Can you work these out from the model? Positions are in its coordinate system, mm. A direction names the side the tool comes from. Coordinates: 2 decimals unless noted, no trailing zeros. Order: outer loops, then holes, each group sorted by start corner. A loop starts at its lowest first (then second) coordinate and runs counter-clockwise, first axis right, second up. Notation, with made-up numbers: (57.5, 79) -> (102.5, 79) arc R35 ccw to (102.5, 111) -> close; hole circle Ø11 at (-24.75, 86). An arc over 180 degrees is marked (long way). Write item = value, one per line.
```python
from build123d import *

# Parameters (mm, degrees)
SKETCH1_W           = 76.2
SKETCH1_H           = 25.4
SKETCH1_W_2         = 70.104
SKETCH1_H_2         = 19.304
BOSS_EXTRUDE1_DEPTH = 200
SKETCH3_W           = 76.2
SKETCH3_H           = 25.4
SKETCH3_W_2         = 70.104
SKETCH3_H_2         = 19.304
BOSS_EXTRUDE2_DEPTH = 38.1
CUT_EXTRUDE1_DEPTH  = 77.2
CUT_EXTRUDE2_START  = 13.832764
SKETCH6_R           = 38.1
CUT_EXTRUDE2_DEPTH  = 83.124802


with BuildPart() as part:
    # Sketch1 → Boss-Extrude1 (new body)
    with BuildSketch(Plane(origin=(0, 0, 0), x_dir=(1, 0, 0), z_dir=(0, 1, 0))):
        Rectangle(SKETCH1_W, SKETCH1_H)
        Rectangle(SKETCH1_W_2, SKETCH1_H_2, mode=Mode.SUBTRACT)
    extrude(amount=BOSS_EXTRUDE1_DEPTH)

    # Sketch3 → Boss-Extrude2 (add)
    with BuildSketch(Plane.XZ):
        Rectangle(SKETCH3_W, SKETCH3_H)
        Rectangle(SKETCH3_W_2, SKETCH3_H_2, mode=Mode.SUBTRACT)
    extrude(amount=BOSS_EXTRUDE2_DEPTH)

    # Sketch5 → Cut-Extrude1 (cut, through all)
    with BuildSketch(Plane(origin=(38.1, 0, 0), x_dir=(0, 0, -1), z_dir=(1, 0, 0))):
        Polygon((-27.756394936, -43.348459281), (21.22080401, -61.959922544), (71.342880626, -33.096384918), (0, 0), (-29.237931348, 13.563649542), align=None)
    extrude(amount=-CUT_EXTRUDE1_DEPTH, mode=Mode.SUBTRACT)

    # Sketch6 → Cut-Extrude2 (cut)
    with BuildSketch(Plane(origin=(56.875227758, 193.523427606, 7.656864493), x_dir=(-0.131571603, 0.016382038, 0.991171298), z_dir=(-0.984807753, 0.112143352, -0.132580384)).offset(CUT_EXTRUDE2_START)):
        Circle(SKETCH6_R)
    extrude(amount=CUT_EXTRUDE2_DEPTH, mode=Mode.SUBTRACT)


solid = part.part
```
Item 1: If I drill on probe 1 along X at (y, z) = (139.5, 5.25); probe 2 along Z at (x, y) = (-12.5, 36.5); probe 3 along Z at (x, y) = (25, 5), over which ranges is the centre line in solid material (lowest first)?
A:
probe_1 = -38.1 to -35.05, 35.05 to 38.1
probe_2 = -12.7 to -9.65, 9.65 to 12.7
probe_3 = -12.7 to -9.65, 9.65 to 10.78
Item 2: I want a section at A-A, the plane y = 122.5. Please give me the cut outline in (x, z).
A:
outline = (-38.1, -12.7) -> (38.1, -12.7) -> (38.1, 12.7) -> (-38.1, 12.7) -> close; hole (-35.05, -9.65) -> (35.05, -9.65) -> (35.05, 9.65) -> (-35.05, 9.65) -> close
Item 3: If we mould it in two halves opening along Z, with no side actions, what happens to faces 3 (the flat face through (-1, 82, -12.7)), 4 (the flat face through (38.1, 79, 0)), 5 (the flat face through (-35.052, 83, 0))? For each: pulls with the +Z half, pulls with the -Z half, needs draft (parallel to the pull), parting line crosses it, or undercut.
A:
face_3 = pulls with the -Z half
face_4 = needs draft
face_5 = undercut
Item 4: I'm going to push a flat-ended pin straight in: P1, Ø12, axis at x = -16, z = -5, coming from the -Y side. Where does the tip first touch, or does it pass through?
A:
P1 = -5.1
Item 5: For faces 1 (the flat face through (35.052, 79, 0)), 2 (the flat face through (-38.1, 83, 0)), which set-ups out of +Z, -Z, +X, -X, +Y, -Y let a thin tool reach every point of the face, with its end or its side?
A:
face_1 = +Y, -Y
face_2 = +Z, -Z, -X, +Y, -Y
